The listing builds one solid part. Answer for the finished solid, in the listing's coordinates (mm). Face numbers are marked on the shaded views. A direction names the side the tool comes from. Coordinates: 2 decimals unless noted, no trailing zeros. Order: outer loops, then holes, each group sorted by start corner. A loop starts at its lowest first (then second) coordinate and runs counter-clockwise, first axis right, second up. Notation, with made-up numbers: (-28, 20) - (-6, 20) arc R16 cw to (-6, 39) - close; hole circle Ø4 at (31, -40). An arc over 180 degrees is marked (long way). Use one line per item in the form item = value. Start each with the question number.
Item 1: Section A-A, the plane z = -8 is taken. Write down the section's boundary in (x, y), and give its area (3 significant figures).
Item 2: Section B-B, the plane z = 9.25 is taken. Write down the section's boundary in (x, y).
Item 3: A tool of negligible diameter and unlimited length cuts with its end or side. For the marked faces 1 and 2, from which of +Z, -Z, +X, -X, +Y, -Y can it reach the whole face along a straight path? Write none if from no direction.
Item 4: Consider line 1 along Y through (x, z) = (0, -12.75); line 2 along X through (y, z) = (-0.05, -9.5). Determine where each line is inside the solid, lowest interval first. Write a range as [from, to].
Item 5: Each of these flat-tipped pins is pushed along its axis until it touches: pin 1 Ø1.5 at (x, y) = (1.5, 1.5) entering from +Z; pin 2 Ø1.2 at (x, y) = (0.5, 0.5) entering from -Z; pin 3 Ø1.7 at (x, y) = (0, 0) entering from -Z. Where does it stop, or does it pass through?
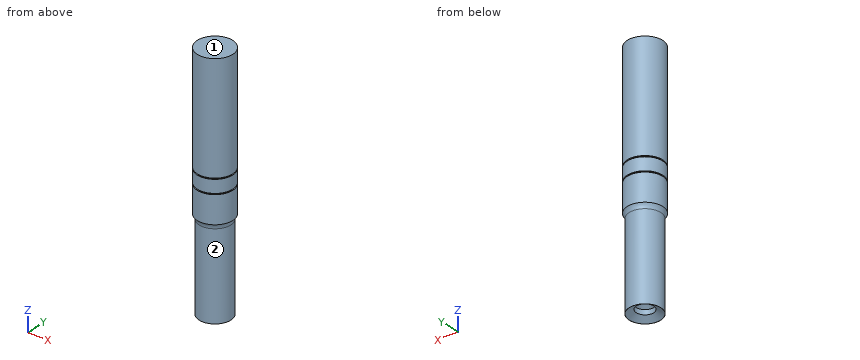
from build123d import *

# Parameters (mm, degrees)
REDONDEO1_R                      = 0.762
TALADRO_DE_MARGEN_PARA_101_D     = 1.9304
TALADRO_DE_MARGEN_PARA_101_DEPTH = 0.9906
TALADRO_DE_MARGEN_PARA_101_TIP   = 0.579950669
CHAFL_N1_SIZE                    = 0.79375
CHAFL_N1_SIZE2                   = 0.458271776


with BuildPart() as part:
    # Croquis1 → Revolución1 (revolve)
    with BuildSketch(Plane(origin=(0, 0, 0), x_dir=(0, 0, -1), z_dir=(1, 0, 0)), mode=Mode.PRIVATE) as revoluci_n1_sk:
        Polygon((-13.4874, 0), (-13.4874, 1.9812), (-1.397, 1.9812), (-1.397, 1.8542), (-1.27, 1.8542), (-1.27, 1.9812), (0.1524, 1.9812), (0.1524, 1.8542), (0.2794, 1.8542), (0.2794, 1.9812), (3.3274, 1.9812), (3.3274, 1.7653), (13.4874, 1.7653), (13.4874, 0), align=None)
    revolve(revoluci_n1_sk.sketch.rotate(Axis((0, 0, 127), (0, 0, -1)), 90), axis=Axis((0, 0, 127), (0, 0, -1)))

    # Redondeo1
    # the kernel refuses this fillet: 0.762 mm, written as the material it adds along each edge
    with BuildSketch(Plane(origin=(0, 0, -3.3274), x_dir=(1, 0, 0), z_dir=(0, 1, 0))) as redondeo1_piece_1:
        with BuildLine():
            CenterArc((2.5273, 0.531430889), REDONDEO1_R, 180, 44.220044428)
            Line((1.7653, 0.531430889), (1.75006, 0.531430889))
            Line((1.75006, 0.531430889), (1.75006, 0))
            Line((1.75006, 0), (1.7653, -0.01524))
            ThreePointArc((1.7653, -0.01524), (1.87325, -0.01524), (1.970278, -0.010628618))
            Line((1.970278, -0.010628618), (1.9812, 0))
        make_face()
    revolve(axis=Axis((0, 0, -3.3274), (0, 0, -1)))

    # Taladro de margen para #101
    with Locations(Plane(origin=(0, 0, -13.4874), x_dir=(-1, 0, 0), z_dir=(0, 0, -1))):
        with Locations((0, 0)):
            Hole(TALADRO_DE_MARGEN_PARA_101_D / 2, depth=TALADRO_DE_MARGEN_PARA_101_DEPTH)
            with Locations((0, 0, -(TALADRO_DE_MARGEN_PARA_101_DEPTH + TALADRO_DE_MARGEN_PARA_101_TIP / 2))):  # 118° drill point
                Cone(0, TALADRO_DE_MARGEN_PARA_101_D / 2, TALADRO_DE_MARGEN_PARA_101_TIP, mode=Mode.SUBTRACT)

    # Chaflán1
    chafl_n1_edges = [part.edges().sort_by_distance(p)[0] for p in [
        (-0.9652, 0, -13.4874),
    ]]
    chafl_n1_side = [part.faces().sort_by_distance(p)[0] for p in [
        (-1.715369776, 0, -13.4874),
    ]]
    chamfer(chafl_n1_edges, length=CHAFL_N1_SIZE, length2=CHAFL_N1_SIZE2, reference=chafl_n1_side[0])


solid = part.part
Response:
q1.outline = circle Ø3.53 at (0, 0)
q1.area = 9.79 mm2
q2.outline = circle Ø3.96 at (0, 0)
q3.face_1 = +Z, +X, -X, +Y, -Y
q3.face_2 = -Z
q4.line_1 = [-1.77, -0.97], [0.97, 1.77]
q4.line_2 = [-1.76, 1.76]
q5.pin_1 = 13.49
q5.pin_2 = -13.23
q5.pin_3 = -12.43
